Here's how the part is built. I have some questions about the finished solid (model axes, mm). Face numbers are marked on the shaded views. A direction names the side the tool comes from. Coordinates: 2 decimals unless noted, no trailing zeros. Write each loop counter-clockwise with the first axis right and the second up, starting at its lowest first coordinate (ties: lowest second). Pieces come first, ordered by that corner, then holes.
Item 1: I want a section at B-B (x = 0). Please give me the cut outline in (y, z), and give its area (3 significant figures).
Item 2: I'm going to push flat-ended pins straight in: P1, Ø3, axis at x = 0.5, y = 6, coming from the +Z side; P2, Ø0.5, axis at y = 2.5, z = -5.5, coming from the +X side; P3, Ø1.5, axis at y = 6, z = -7, coming from the +X side; P4, Ø8, axis at x = 0, z = 0, coming from the +Y side. Where does each tip first touch, or does it pass through?
Item 3: I want a section at A-A (z = 0). Please give me the cut outline in (x, y), and give its area (3 significant figures).
Item 4: I want a section at C-C (y = 1.75). Please give me the cut outline in (x, z), and give its area (3 significant figures).
Item 5: Please list where these lines run through material, in increasing order: line 1 (X direction, y = 4, z = 0); line 2 (X direction, y = 4, z = -5); line 3 (Y direction, x = -3, z = -9.75).
Item 6: For the marked faces 4, 5 and 6, which set-ups out of +Z, -Z, +X, -X, +Y, -Y let a thin tool reach every point of the face, with its end or its side?
Item 7: I want a section at D-D (x = -3). Please give me the cut outline in (y, z).
Item 8: If we mould it in two halves opening along Z, with no side actions, what happens to the marked faces 1, 2 and 3? For each: pulls with the +Z half, pulls with the -Z half, needs draft (parallel to the pull), parting line crosses it, or undercut.
from build123d import *

# Parameters (mm, degrees)
SKETCH1_R           = 9.5
BOSS_EXTRUDE1_DEPTH = 10
SKETCH2_R           = 12
BOSS_EXTRUDE2_DEPTH = 2.5
CUT_EXTRUDE2_DEPTH  = 2.5
SKETCH5_R           = 1.75
CUT_EXTRUDE3_DEPTH  = 15


with BuildPart() as part:
    # Sketch1 → Boss-Extrude1 (new body)
    with BuildSketch(Plane(origin=(0, 0, 0), x_dir=(1, 0, 0), z_dir=(0, 1, 0))):
        Circle(SKETCH1_R)
        with BuildLine():
            Line((-1.332, 6.504006227), (-1.332, 4.704006227))
            Line((-1.332, 4.704006227), (1.33, 4.704006227))
            Line((1.33, 4.704006227), (1.33, 6.5044155))
            ThreePointArc((1.33, 6.5044155), (0.001020723, -6.638999922), (-1.332, 6.504006227))
        make_face(mode=Mode.SUBTRACT)
    extrude(amount=BOSS_EXTRUDE1_DEPTH)

    # Sketch2 → Boss-Extrude2 (add)
    with BuildSketch(Plane.XZ):
        Circle(SKETCH2_R)
    extrude(amount=-BOSS_EXTRUDE2_DEPTH)

    # Sketch4 → Cut-Extrude2 (cut)
    with BuildSketch(Plane(origin=(0, 2.5, 0), x_dir=(1, 0, 0), z_dir=(0, 1, 0))):
        with BuildLine():
            Line((-1.332, 4.704006227), (1.33, 4.704006227))
            Line((1.33, 4.704006227), (1.33, 6.5044155))
            ThreePointArc((1.33, 6.5044155), (0.001020723, -6.638999922), (-1.332, 6.504006227))
            Line((-1.332, 6.504006227), (-1.332, 4.704006227))
        make_face()
    extrude(amount=-CUT_EXTRUDE2_DEPTH, mode=Mode.SUBTRACT)

    # Sketch5 → Cut-Extrude3 (cut)
    with BuildSketch(Plane.XY.offset(-4.704006227)):
        with Locations((-0.000110737, 6.499999939)):
            Circle(SKETCH5_R)
    extrude(amount=CUT_EXTRUDE3_DEPTH, mode=Mode.SUBTRACT)


solid = part.part
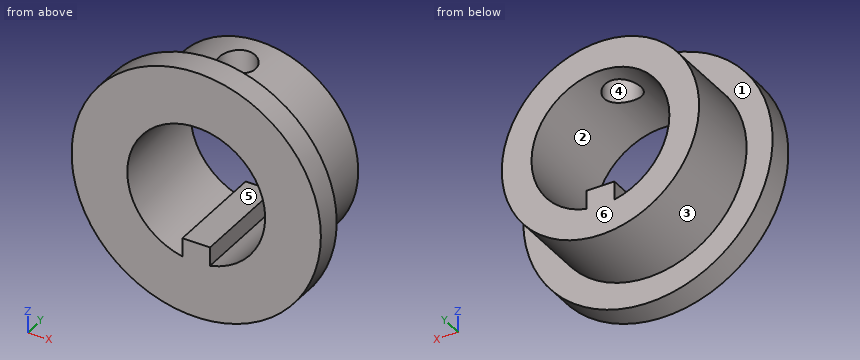
Answer:
1. outline: (0, -12) - (2.5, -12) - (2.5, -9.5) - (10, -9.5) - (10, -4.7) - (0, -4.7) - close; (0, 6.64) - (4.75, 6.64) - (4.75, 9.5) - (2.5, 9.5) - (2.5, 12) - (0, 12) - close; (8.25, 6.64) - (10, 6.64) - (10, 9.5) - (8.25, 9.5) - close
1. area: 79.1 mm2
2. P1: stops at z = 9.5
2. P2: stops at x = 10.79
2. P3: stops at x = 7.15
2. P4: passes through
3. outline: (-12, 0) - (-6.64, 0) - (-6.64, 10) - (-9.5, 10) - (-9.5, 2.5) - (-12, 2.5) - close; (6.64, 0) - (12, 0) - (12, 2.5) - (9.5, 2.5) - (9.5, 10) - (6.64, 10) - close
3. area: 69.7 mm2
4. outline: circle Ø24 at (0, 0); hole (-1.33, -6.5) - (-1.33, -4.7) - (1.33, -4.7) - (1.33, -6.5) arc R6.64 ccw (long way) to start
4. area: 319 mm2
5. line 1: x = -9.5 to -6.64, 6.64 to 9.5
5. line 2: x = -8.08 to -4.37, -1.33 to 1.33, 4.37 to 8.08
5. line 3: y = 0 to 2.5
6. face 4: +Z
6. face 5: +Y, -Y
6. face 6: +Z, -Z, +X, -X, +Y
7. outline: (0, -11.62) - (2.5, -11.62) - (2.5, -9.01) - (10, -9.01) - (10, -5.92) - (0, -5.92) - close; (0, 5.92) - (10, 5.92) - (10, 9.01) - (2.5, 9.01) - (2.5, 11.62) - (0, 11.62) - close
8. face 1: needs draft
8. face 2: undercut
8. face 3: parting line crosses it
